Study the drawing (mm; zero at the part's minimum x, y, z) and answer. A direction names the side the tool comes from. Round coordinates to 2 decimals unless told otherwise and drop trailing zeros. Write each loop counter-clockwise with the first axis right and the second up, starting at its lowest first coordinate (ties: lowest second). Pieces come first, ordered by that corner, then holes.
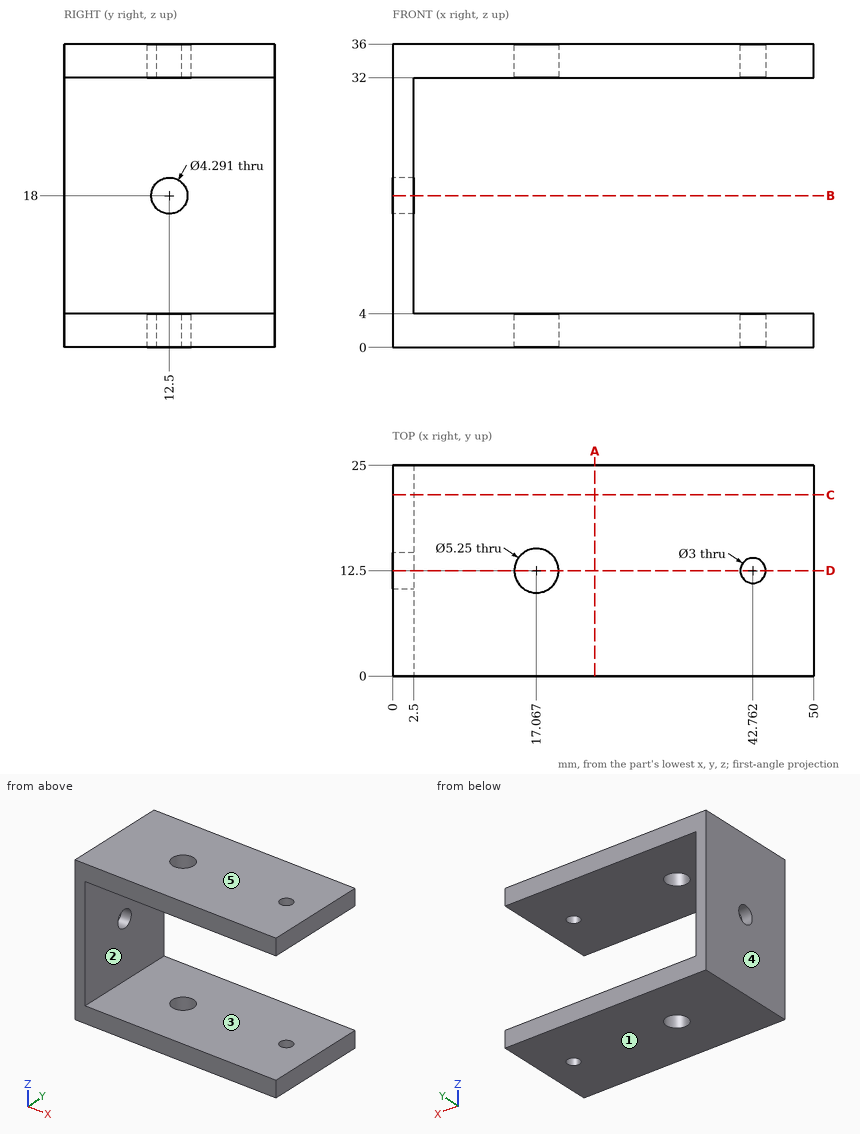
1. For a pull along Z with two mould halves and no side action, classify the marked faces 3, 4 and 5 as released by +Z, released by -Z, zero draft, split by the parting line, or undercut.
Geometry says:
face 3: undercut
face 4: zero draft
face 5: released by +Z
2. Section B-B on z = 18 is taken. Determine the outline of the cut face in (x, y) (1 decimal).
Geometry says:
outline: (0, 0) - (2.5, 0) - (2.5, 10.4) - (0, 10.4) - close; (0, 14.6) - (2.5, 14.6) - (2.5, 25) - (0, 25) - close
3. Section D-D on y = 12.5 is taken. Determine the outline of the cut face in (x, z) (1 decimal).
Geometry says:
outline: (0, 0) - (14.4, 0) - (14.4, 4) - (2.5, 4) - (2.5, 15.9) - (0, 15.9) - close; (0, 20.1) - (2.5, 20.1) - (2.5, 32) - (14.4, 32) - (14.4, 36) - (0, 36) - close; (19.7, 0) - (41.3, 0) - (41.3, 4) - (19.7, 4) - close; (19.7, 32) - (41.3, 32) - (41.3, 36) - (19.7, 36) - close; (44.3, 0) - (50, 0) - (50, 4) - (44.3, 4) - close; (44.3, 32) - (50, 32) - (50, 36) - (44.3, 36) - close
4. Given pin 1 (7.5 mm diameter, centred on y = 10.5, z = 16, fed in from +X), flat-ended and moving along its own axis, determine where the tip first touches the part or whether it passes through.
Geometry says:
pin 1: stops at x = 2.5
5. A tool of negligible diameter and unlimited length cuts with its end or side. For the marked faces 1 and 2, from which of +Z, -Z, +X, -X, +Y, -Y can it reach the whole face along a straight path? Write none if from no direction.
Geometry says:
face 1: -Z, +X, -X, +Y, -Y
face 2: +X, +Y, -Y
6. Straight lines are drawn through the part: line 1 along Z through (x, y) = (40, 4); line 2 along X through (y, z) = (4.5, 24). For each, find the intervals that lie inside material, in ascending order.
Geometry says:
line 1: z = 0 to 4, 32 to 36
line 2: x = 0 to 2.5
7. Section A-A on x = 24 is taken. Determine the outline of the cut face in (y, z).
Geometry says:
outline: (0, 0) - (25, 0) - (25, 4) - (0, 4) - close; (0, 32) - (25, 32) - (25, 36) - (0, 36) - close
8. Section C-C on y = 21.5 is taken. Determine the outline of the cut face in (x, z), plus the area to 3 significant figures.
Geometry says:
outline: (0, 0) - (50, 0) - (50, 4) - (2.5, 4) - (2.5, 32) - (50, 32) - (50, 36) - (0, 36) - close
area: 470 mm2
